Build history of the part. All positions in model axes, mm. A direction names the side the tool comes from. Give positions to 0.01 mm unless a question says otherwise; leave off trailing zeros. Order: outer loops, then holes, each group sorted by start corner. A loop starts at its lowest first (then second) coordinate and runs counter-clockwise, first axis right, second up. Notation, with made-up numbers: (-17, -26.5) - (26, -26.5) arc R24 ccw to (26, -7.5) - close; hole circle Ø11 at (0.5, -30). An arc over 180 degrees is marked (long way). Use a Markdown table: item, result.
from build123d import *

# Parameters (mm, degrees)
SKETCH_1_W      = 22
SKETCH_1_H      = 10
EXTRUDE_1_DEPTH = 8
SKETCH_2_R      = 1.1
EXTRUDE_2_DEPTH = 1.6


with BuildPart() as part:
    # 草图1 → 凸台-拉伸1 (new body)
    with BuildSketch(Plane.XY):
        with Locations((11, 5)):
            Rectangle(SKETCH_1_W, SKETCH_1_H)
    extrude(amount=EXTRUDE_1_DEPTH)

    # 草图2 → 凸台-拉伸2 (add)
    with BuildSketch(Plane.XY.offset(8)):
        Polygon((0, 7), (-4, 7), (-4, 3), (0, 3), (0, 0), (22, 0), (22, 3), (26, 3), (26, 7), (22, 7), (22, 10), (0, 10), align=None)
        with Locations((-2, 5)):
            Circle(SKETCH_2_R, mode=Mode.SUBTRACT)
        with Locations((24, 5)):
            Circle(SKETCH_2_R, mode=Mode.SUBTRACT)
    extrude(amount=EXTRUDE_2_DEPTH)


solid = part.part
1) Slice it at A-A (y = 5). Write the cut outline in (x, z).
Computed:
| item | result |
|---|---|
| outline | (-4, 8) - (-3.1, 8) - (-3.1, 9.6) - (-4, 9.6) - close; (-0.9, 8) - (0, 8) - (0, 0) - (22, 0) - (22, 8) - (22.9, 8) - (22.9, 9.6) - (-0.9, 9.6) - close; (25.1, 8) - (26, 8) - (26, 9.6) - (25.1, 9.6) - close |
2) Pin check, flat tips, straight feed: P1, Ø1.8, axis at x = -3, z = 9, coming from the -Y side; P2, Ø2, axis at y = 8, z = 5, coming from the +X side; P3, Ø1.8, axis at x = -2, z = 9, coming from the +Y side. Stop position of each tip, or through.
Computed:
| item | result |
|---|---|
| P1 | stops at y = 3 |
| P2 | stops at x = 22 |
| P3 | stops at y = 7 |
3) Slice it at D-D (y = 0.75). Write the cut outline in (x, z).
Computed:
| item | result |
|---|---|
| outline | (0, 0) - (22, 0) - (22, 9.6) - (0, 9.6) - close |
4) Two-plate mould, pull along Y, no slides. Class faces 4 (the flat face through (24, 3, 9)), 5 (the flat face through (-3, 6, 8)), 6 (the cylindrical face through (-0.95, 5.33, 8.79)): +Y half, -Y half, draft (parallel to the pull), parting line (faces both ways), or undercut.
Computed:
| item | result |
|---|---|
| face 4 | -Y half |
| face 5 | draft |
| face 6 | undercut |
5) Wall check: line 1 (Y direction, x = -2, z = 8.4); line 2 (Z direction, x = 24, y = 6.75); line 3 (X direction, y = 3.5, z = 7). Give the ranges that are in metal, low to high. Write a range as from..to.
Computed:
| item | result |
|---|---|
| line 1 | y = 3..3.9, 6.1..7 |
| line 2 | z = 8..9.6 |
| line 3 | x = 0..22 |
6) Slice it at C-C (z = 9.25). Write the cut outline in (x, y), and give its area (3 significant figures).
Computed:
| item | result |
|---|---|
| outline | (-4, 3) - (0, 3) - (0, 0) - (22, 0) - (22, 3) - (26, 3) - (26, 7) - (22, 7) - (22, 10) - (0, 10) - (0, 7) - (-4, 7) - close; hole circle Ø2.2 at (-2, 5); hole circle Ø2.2 at (24, 5) |
| area | 244 mm² |
7) Slice it at B-B (x = 24). Write the cut outline in (y, z), and give its area (3 significant figures).
Computed:
| item | result |
|---|---|
| outline | (3, 8) - (3.9, 8) - (3.9, 9.6) - (3, 9.6) - close; (6.1, 8) - (7, 8) - (7, 9.6) - (6.1, 9.6) - close |
| area | 2.88 mm² |
8) Tool access for faces 1 (the flat face through (24, 7, 9)), 2 (the flat face through (23, 6, 8)), 3 (the flat face through (-2, 3, 9)): list every direction of +Z, -Z, +X, -X, +Y, -Y with a clear straight run to the whole face (end or side of a thin tool).
Computed:
| item | result |
|---|---|
| face 1 | +Z, -Z, +X, +Y |
| face 2 | -Z, +X, +Y, -Y |
| face 3 | +Z, -Z, -X, -Y |
